from build123d import *

# Parameters (mm, degrees)
ESQUISSE1_W             = 230
ESQUISSE1_H             = 230
BOSS_EXTRU_1_DEPTH      = 53
ESQUISSE2_W             = 220
ESQUISSE2_H             = 220
ENL_V_MAT_EXTRU_1_DEPTH = 50
ESQUISSE3_W             = 226
ESQUISSE3_H             = 226
ENL_V_MAT_EXTRU_2_DEPTH = 3
ESQUISSE4_R             = 12.5
ENL_V_MAT_EXTRU_3_DEPTH = 13
ESQUISSE5_R             = 1.25
ENL_V_MAT_EXTRU_4_DEPTH = 13
ESQUISSE6_W             = 26.976344154
ESQUISSE6_H             = 1.5
ESQUISSE6_W_2           = 27.280131813
ESQUISSE6_W_3           = 27.280131814
BOSS_EXTRU_2_DEPTH      = 5
ESQUISSE7_R             = 3
ENL_V_MAT_EXTRU_5_DEPTH = 5
ESQUISSE9_W             = 12.6
ESQUISSE9_H             = 11.4
ENL_V_MAT_EXTRU_6_DEPTH = 5
ESQUISSE10_R            = 1.5
ESQUISSE10_R_2          = 2
ESQUISSE10_R_3          = 2.5
ESQUISSE10_R_4          = 3
ENL_V_MAT_EXTRU_7_DEPTH = 10


with BuildPart() as part:
    # Esquisse1 → Boss.-Extru.1 (new body)
    with BuildSketch(Plane(origin=(0, 0, 0), x_dir=(1, 0, 0), z_dir=(0, 1, 0))):
        with Locations((115, 115)):
            Rectangle(ESQUISSE1_W, ESQUISSE1_H)
    extrude(amount=BOSS_EXTRU_1_DEPTH)

    # Esquisse2 → Enlèv. mat.-Extru.1 (cut)
    with BuildSketch(Plane(origin=(0, 53, 0), x_dir=(1, 0, 0), z_dir=(0, 1, 0))):
        with Locations((115, 115)):
            Rectangle(ESQUISSE2_W, ESQUISSE2_H)
    extrude(amount=-ENL_V_MAT_EXTRU_1_DEPTH, mode=Mode.SUBTRACT)

    # Esquisse3 → Enlèv. mat.-Extru.2 (cut)
    with BuildSketch(Plane(origin=(0, 53, 0), x_dir=(1, 0, 0), z_dir=(0, 1, 0))):
        with Locations((115, 115)):
            Rectangle(ESQUISSE3_W, ESQUISSE3_H)
    extrude(amount=-ENL_V_MAT_EXTRU_2_DEPTH, mode=Mode.SUBTRACT)

    # Esquisse4 → Enlèv. mat.-Extru.3 (cut)
    with BuildSketch(Plane(origin=(0, 0, -230), x_dir=(-1, 0, 0), z_dir=(0, 0, -1))):
        with Locations((-30, 26.5)):
            Circle(ESQUISSE4_R)
    extrude(amount=-ENL_V_MAT_EXTRU_3_DEPTH, mode=Mode.SUBTRACT)

    # Esquisse5 → Enlèv. mat.-Extru.4 (cut)
    with BuildSketch(Plane(origin=(0, 0, -230), x_dir=(-1, 0, 0), z_dir=(0, 0, -1))):
        with Locations((-40, 36.5)):
            Circle(ESQUISSE5_R)
        with Locations((-20, 36.5)):
            Circle(ESQUISSE5_R)
        with Locations((-20, 16.5)):
            Circle(ESQUISSE5_R)
        with Locations((-40, 16.5)):
            Circle(ESQUISSE5_R)
    extrude(amount=-ENL_V_MAT_EXTRU_4_DEPTH, mode=Mode.SUBTRACT)

    # Esquisse6 → Boss.-Extru.2 (add)
    with BuildSketch(Plane(origin=(0, 0, -230), x_dir=(-1, 0, 0), z_dir=(0, 0, -1))):
        with Locations((-29.668195525, 26.5)):
            Rectangle(ESQUISSE6_W, ESQUISSE6_H)
        with Locations((-29.516301696, 31)):
            Rectangle(ESQUISSE6_W_2, ESQUISSE6_H)
        with BuildLine():
            Line((-39.807522623, 18.75), (-20.192477377, 18.75))
            add(Edge.make_bspline(
                [(-20.192477377, 18.75), (-20.3726905, 17.550508754), (-21.59241414, 17.25)],
                knots=[0, 0, 0, 1, 1, 1], degree=2))
            Line((-21.59241414, 17.25), (-38.40758586, 17.25))
            add(Edge.make_bspline(
                [(-39.807522623, 18.75), (-39.455191276, 17.680066298), (-38.40758586, 17.25)],
                knots=[0, 0, 0, 1, 1, 1], degree=2))
        make_face()
        with Locations((-29.303650334, 22)):
            Rectangle(ESQUISSE6_W_3, ESQUISSE6_H)
        with BuildLine():
            Line((-39.807522623, 34.25), (-20.192477377, 34.25))
            add(Edge.make_bspline(
                [(-21.59241414, 35.75), (-20.476912109, 35.349681649), (-20.192477377, 34.25)],
                knots=[0, 0, 0, 1, 1, 1], degree=2))
            Line((-21.59241414, 35.75), (-38.40758586, 35.75))
            add(Edge.make_bspline(
                [(-39.807522623, 34.25), (-39.526090214, 35.47410851), (-38.40758586, 35.75)],
                knots=[0, 0, 0, 1, 1, 1], degree=2))
        make_face()
    extrude(amount=-BOSS_EXTRU_2_DEPTH)

    # Esquisse7 → Enlèv. mat.-Extru.5 (cut)
    with BuildSketch(Plane(origin=(0, 0, -230), x_dir=(-1, 0, 0), z_dir=(0, 0, -1))):
        with Locations((-215, 8)):
            Circle(ESQUISSE7_R)
    extrude(amount=-ENL_V_MAT_EXTRU_5_DEPTH, mode=Mode.SUBTRACT)

    # Esquisse9 → Enlèv. mat.-Extru.6 (cut)
    with BuildSketch(Plane(origin=(0, 0, -230), x_dir=(-1, 0, 0), z_dir=(0, 0, -1))):
        with Locations((-193.7, 10.836521705)):
            Rectangle(ESQUISSE9_W, ESQUISSE9_H)
    extrude(amount=-ENL_V_MAT_EXTRU_6_DEPTH, mode=Mode.SUBTRACT)

    # Esquisse10 → Enlèv. mat.-Extru.7 (cut)
    with BuildSketch(Plane(origin=(0, 0, -230), x_dir=(-1, 0, 0), z_dir=(0, 0, -1))):
        with Locations((-152.831654842, 9.359863556)):
            Circle(ESQUISSE10_R)
        with Locations((-142.831654842, 9.359863556)):
            Circle(ESQUISSE10_R_2)
        with Locations((-132.831654842, 9.359863556)):
            Circle(ESQUISSE10_R_3)
        with Locations((-122.831654842, 9.359863556)):
            Circle(ESQUISSE10_R_4)
        with Locations((-112.831654842, 9.359863556)):
            Circle(ESQUISSE10_R_3)
        with Locations((-102.831654842, 9.359863556)):
            Circle(ESQUISSE10_R_2)
        with Locations((-92.831654842, 9.359863556)):
            Circle(ESQUISSE10_R)
    extrude(amount=-ENL_V_MAT_EXTRU_7_DEPTH, mode=Mode.SUBTRACT)


solid = part.part
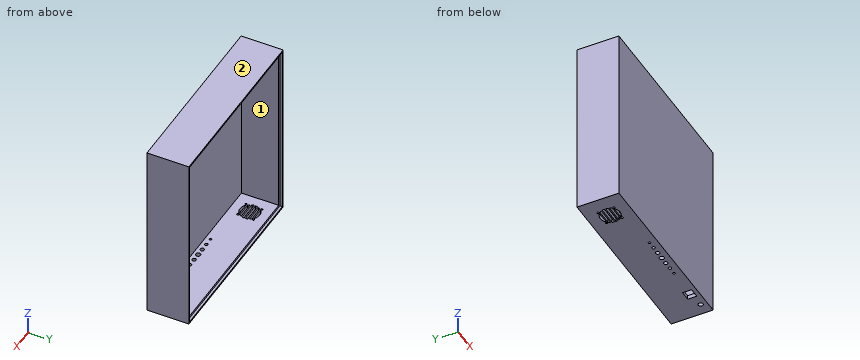
Can you work these out from the model? Positions are in its coordinate system, mm. Face numbers are marked on the shaded views. A direction names the side the tool comes from. Give positions to 0.01 mm unless a question says otherwise; leave off trailing zeros. Write each loop counter-clockwise with the first axis right and the second up, starting at its lowest first coordinate (ties: lowest second). Pieces come first, ordered by that corner, then holes. Notation, with made-up numbers: (55.25, 85.5) -> (61.25, 85.5) arc R30 cw to (61.25, 113.5) -> close; hole circle Ø5 at (53, 8). An arc over 180 degrees is marked (long way). Answer as a JSON object with one key per item and string values. Group by question number.
Item 1: Please list where these lines run through material, in increasing order: line 1 (X direction, y = 40, z = -144.5); line 2 (Z direction, x = 203, y = 19.5); line 3 (Y direction, x = 165, z = -46). Write a range as [from, to].
Item 2: Suppose I cut it at B-B (x = 78). Please give me the cut outline in (y, z), plus the area to 3 significant figures.
Item 3: For the marked faces 1 and 2, which set-ups out of +Z, -Z, +X, -X, +Y, -Y let a thin tool reach every point of the face, with its end or its side?
Item 4: Suppose I cut it at D-D (x = 25.5). State how many separate pieces and enclosed holes the cut face has, plus the area to 3 significant figures.
Item 5: I'm going to push flat-ended pins straight in: P1, Ø8, axis at x = 185, y = 22, coming from the +Z side; P2, Ø6, axis at x = 165, z = -201, coming from the +Y side; P3, Ø3, axis at x = 132.83, y = 9.36, coming from the -Z side. Where does each tip first touch, or does it pass through?
Item 6: Suppose I cut it at C-C (z = -30.5). Please give me the cut outline in (x, y), plus the area to 3 significant figures.
Item 7: Suppose I cut it at A-A (x = 215). Please give me the cut outline in (y, z).
Findings:
{
 "1": {"line 1": "x = [0, 5], [225, 230]", "line 2": "z = [-230, -225], [-5, 0]", "line 3": "y = [0, 3]"},
 "2": {"outline": "(0, -230) -> (53, -230) -> (53, -228) -> (50, -228) -> (50, -225) -> (3, -225) -> (3, -5) -> (50, -5) -> (50, -2) -> (53, -2) -> (53, 0) -> (0, 0) -> close", "area": "1,170 mm²"},
 "3": {"face 1": "+Y", "face 2": "+Z, +X, -X, +Y, -Y"},
 "4": {"separate pieces": "7", "enclosed holes": "0", "area": "1,090 mm²"},
 "5": {"P1": "stops at z = 0", "P2": "stops at y = 3", "P3": "stops at z = -5"},
 "6": {"outline": "(0, 0) -> (230, 0) -> (230, 53) -> (228, 53) -> (228, 50) -> (225, 50) -> (225, 3) -> (5, 3) -> (5, 50) -> (2, 50) -> (2, 53) -> (0, 53) -> close", "area": "1,170 mm²"},
 "7": {"outline": "(0, -230) -> (5, -230) -> (5, -225) -> (3, -225) -> (3, -5) -> (50, -5) -> (50, -2) -> (53, -2) -> (53, 0) -> (0, 0) -> close; (11, -230) -> (53, -230) -> (53, -228) -> (50, -228) -> (50, -225) -> (11, -225) -> close"}
}
